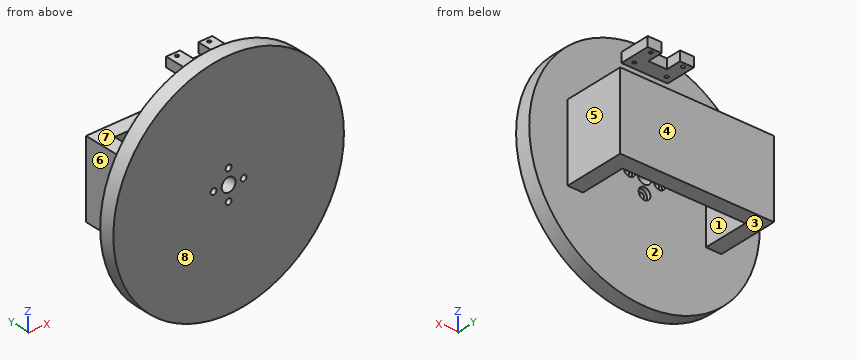
from build123d import *

# Parameters (mm, degrees)
SKETCH1_R           = 75
BOSS_EXTRUDE1_DEPTH = 10
SKETCH2_R           = 1.905
CUT_EXTRUDE2_DEPTH  = 11
CIRPATTERN1_COUNT   = 4
SKETCH3_R           = 4.5
CUT_EXTRUDE3_DEPTH  = 11
SKETCH4_R           = 3.81
CUT_EXTRUDE4_DEPTH  = 2.54
CIRPATTERN2_COUNT   = 4
SKETCH5_W           = 10
SKETCH5_H           = 50
BOSS_EXTRUDE2_DEPTH = 40
SKETCH6_W           = 50
SKETCH6_H           = 10
BOSS_EXTRUDE3_DEPTH = 40
SKETCH7_W           = 30
SKETCH7_H           = 6.35
BOSS_EXTRUDE4_DEPTH = 20
CUT_EXTRUDE5_REACH  = 143.35
SKETCH8_R           = 1.1
SKETCH8_W           = 12
SKETCH8_H           = 20


with BuildPart() as part:
    # Sketch1 → Boss-Extrude1 (new body)
    with BuildSketch(Plane(origin=(0, 0, 0), x_dir=(1, 0, 0), z_dir=(0, 1, 0))):
        Circle(SKETCH1_R)
    extrude(amount=BOSS_EXTRUDE1_DEPTH)

    # Sketch2 → Cut-Extrude2 (cut, through all)
    with BuildSketch(Plane(origin=(0, 10, 0), x_dir=(1, 0, 0), z_dir=(0, 1, 0))):
        with Locations((0, 9.779)):
            Circle(SKETCH2_R)
    cut_extrude2 = extrude(amount=-CUT_EXTRUDE2_DEPTH, mode=Mode.SUBTRACT)

    # CirPattern1: Cut-Extrude2 ×4 about axis
    cirpattern1_axis = Axis((0, 0, 0), (0, 1, 0))
    for i in range(1, CIRPATTERN1_COUNT):
        add(cut_extrude2.rotate(cirpattern1_axis, i * 360 / CIRPATTERN1_COUNT), mode=Mode.SUBTRACT)

    # Sketch3 → Cut-Extrude3 (cut, through all)
    with BuildSketch(Plane(origin=(0, 10, 0), x_dir=(1, 0, 0), z_dir=(0, 1, 0))):
        Circle(SKETCH3_R)
    extrude(amount=-CUT_EXTRUDE3_DEPTH, mode=Mode.SUBTRACT)

    # Sketch4 → Cut-Extrude4 (cut)
    with BuildSketch(Plane(origin=(0, 10, 0), x_dir=(1, 0, 0), z_dir=(0, 1, 0))):
        with Locations((0, 9.779)):
            Circle(SKETCH4_R)
    cut_extrude4 = extrude(amount=-CUT_EXTRUDE4_DEPTH, mode=Mode.SUBTRACT)

    # CirPattern2: Cut-Extrude4 ×4 about axis
    cirpattern2_axis = Axis((0, 0, 0), (0, 1, 0))
    for i in range(1, CIRPATTERN2_COUNT):
        add(cut_extrude4.rotate(cirpattern2_axis, i * 360 / CIRPATTERN2_COUNT), mode=Mode.SUBTRACT)

    # Sketch5 → Boss-Extrude2 (add)
    with BuildSketch(Plane(origin=(0, 10, 0), x_dir=(1, 0, 0), z_dir=(0, 1, 0))):
        with Locations((-45, 0)):
            Rectangle(SKETCH5_W, SKETCH5_H)
    boss_extrude2 = extrude(amount=BOSS_EXTRUDE2_DEPTH)

    # Sketch6 → Boss-Extrude3 (add)
    with BuildSketch(Plane(origin=(-40, 0, 0), x_dir=(0, 0, -1), z_dir=(1, 0, 0))):
        with Locations((0, 45)):
            Rectangle(SKETCH6_W, SKETCH6_H)
    boss_extrude3 = extrude(amount=BOSS_EXTRUDE3_DEPTH)

    # Mirror1: Boss-Extrude2, Boss-Extrude3 across plane
    add(boss_extrude2.mirror(Plane(origin=(0, 0, 0), x_dir=(0, 0, 1), z_dir=(1, 0, 0))))
    add(boss_extrude3.mirror(Plane(origin=(0, 0, 0), x_dir=(0, 0, 1), z_dir=(1, 0, 0))))

    # Sketch7 → Boss-Extrude4 (add)
    with BuildSketch(Plane(origin=(0, 10, 0), x_dir=(1, 0, 0), z_dir=(0, 1, 0))):
        with Locations((0, -63.175)):
            Rectangle(SKETCH7_W, SKETCH7_H)
    extrude(amount=BOSS_EXTRUDE4_DEPTH)

    # Sketch8 → Cut-Extrude5 (cut, up to next)
    with BuildSketch(Plane.XY.offset(66.35), mode=Mode.PRIVATE) as cut_extrude5_sk1:
        with Locations((-10.5, 27)):
            Circle(SKETCH8_R)
    cut_extrude5_tool1 = extrude(cut_extrude5_sk1.sketch, amount=-CUT_EXTRUDE5_REACH, mode=Mode.PRIVATE) & part.part
    add(cut_extrude5_tool1.solids().sort_by_distance((-10.5, 27, 66.35))[0], mode=Mode.SUBTRACT)
    # Sketch8 → Cut-Extrude5 (cut, up to next)
    with BuildSketch(Plane.XY.offset(66.35), mode=Mode.PRIVATE) as cut_extrude5_sk2:
        with Locations((-10.5, 14.5)):
            Circle(SKETCH8_R)
    cut_extrude5_tool2 = extrude(cut_extrude5_sk2.sketch, amount=-CUT_EXTRUDE5_REACH, mode=Mode.PRIVATE) & part.part
    add(cut_extrude5_tool2.solids().sort_by_distance((-10.5, 14.5, 66.35))[0], mode=Mode.SUBTRACT)
    # Sketch8 → Cut-Extrude5 (cut, up to next)
    with BuildSketch(Plane.XY.offset(66.35), mode=Mode.PRIVATE) as cut_extrude5_sk3:
        with Locations((10.5, 27)):
            Circle(SKETCH8_R)
    cut_extrude5_tool3 = extrude(cut_extrude5_sk3.sketch, amount=-CUT_EXTRUDE5_REACH, mode=Mode.PRIVATE) & part.part
    add(cut_extrude5_tool3.solids().sort_by_distance((10.5, 27, 66.35))[0], mode=Mode.SUBTRACT)
    # Sketch8 → Cut-Extrude5 (cut, up to next)
    with BuildSketch(Plane.XY.offset(66.35), mode=Mode.PRIVATE) as cut_extrude5_sk4:
        with Locations((10.5, 14.5)):
            Circle(SKETCH8_R)
    cut_extrude5_tool4 = extrude(cut_extrude5_sk4.sketch, amount=-CUT_EXTRUDE5_REACH, mode=Mode.PRIVATE) & part.part
    add(cut_extrude5_tool4.solids().sort_by_distance((10.5, 14.5, 66.35))[0], mode=Mode.SUBTRACT)
    # Sketch8 → Cut-Extrude5 (cut, up to next)
    with BuildSketch(Plane.XY.offset(66.35), mode=Mode.PRIVATE) as cut_extrude5_sk5:
        with Locations((0, 30)):
            Rectangle(SKETCH8_W, SKETCH8_H)
    cut_extrude5_tool5 = extrude(cut_extrude5_sk5.sketch, amount=-CUT_EXTRUDE5_REACH, mode=Mode.PRIVATE) & part.part
    add(cut_extrude5_tool5.solids().sort_by_distance((0, 30, 66.35))[0], mode=Mode.SUBTRACT)


solid = part.part
For this review, take the finished solid that the model builds, in its own axes (mm). Face numbers are marked on the shaded views. A direction names the side the tool comes from. Round coordinates to 2 decimals unless told otherwise and drop trailing zeros. Loops run counter-clockwise (first coordinate to the right, second up) from the corner with the lowest first, then second, coordinate; pieces in that order, holes last. Notation, with made-up numbers: (-40, 49.5) - (-33, 49.5) arc R17 ccw to (-33, 73.5) - close; hole circle Ø9 at (45, 78). An arc over 180 degrees is marked (long way). Put each result on its own line as item: value. Start each with the question number.
1. Consider section D-D on y = 42. State the section outline as (x, z) points, plus the area to 3 significant figures.
2. Consider section A-A on z = 0. State how many separate pieces and enclosed holes the cut face has, plus the area to 3 significant figures.
3. Insertion check: P1, Ø4, axis at y = 10, z = 58, coming from the -X side; P2, Ø2.5, axis at x = 10.5, y = 14.5, coming from the +Z side; P3, Ø1, axis at x = 36, z = 58, coming from the +Y side; P4, Ø1.3, axis at x = -10.5, y = 27, coming from the -Z side. Each pin has a flat end and moves straight along its axis. Give the tip position at first contact, or say it passes through.
4. For probe 1 along X at (y, z) = (9.2, 0); probe 2 along Z at (x, y) = (0, 4), list the stretches that pass through material, from the lowest coordinate up. Write a range as [from, to].
5. Consider section B-B on y = 32. State the section outline as (x, z) points.
6. Mouldability with a two-part tool opening along Y and no side actions: class the marked faces 1, 2, 3 and 4 as +Y half, -Y half, draft (parallel to the pull), parting line (faces both ways), or undercut.
7. For the marked faces 5, 6, 7 and 8, list the 3-axis set-ups (+Z, -Z, +X, -X, +Y, -Y) from which the entire face can be reached by the end or side of a thin tool; tool diameter is ignored.
Result sheet:
1. outline: (-50, -25) - (50, -25) - (50, 25) - (-50, 25) - close
1. area: 5,000 mm^2
2. separate pieces: 3
2. enclosed holes: 0
2. area: 2,910 mm^2
3. P1: x = -49.89
3. P2: z = 66.35
3. P3: y = 10
3. P4: through
4. probe 1: [-75, -13.59], [-5.97, -4.5], [4.5, 5.97], [13.59, 75]
4. probe 2: [-75, -11.68], [-7.87, -4.5], [4.5, 7.87], [11.68, 75]
5. outline: (-50, -25) - (-40, -25) - (-40, 25) - (-50, 25) - close; (40, -25) - (50, -25) - (50, 25) - (40, 25) - close
6. face 1: undercut
6. face 2: undercut
6. face 3: draft
6. face 4: +Y half
7. face 5: +Z, -Z, +X, +Y
7. face 6: +Z, -Z, -X, +Y
7. face 7: +Z, +X, -X, +Y
7. face 8: +Z, -Z, +X, -X, -Y
